For this review, take the finished solid that the model builds, in its own axes (mm). A direction names the side the tool comes from. Round coordinates to 2 decimals unless told otherwise and drop trailing zeros. Write each loop counter-clockwise with the first axis right and the second up, starting at its lowest first coordinate (ties: lowest second). Pieces come first, ordered by that corner, then holes. Notation, with made-up numbers: (87, 28) - (129, 28) arc R15 cw to (129, 33) - close; hole circle Ø3 at (55, 86). An arc over 180 degrees is marked (long way). Answer in a Markdown table with one row per item. Add a question column.
from build123d import *

# Parameters (mm, degrees)
EXTRUDE_1_DEPTH              = 300
HOLE_WIZARD_M6_1_D           = 6.4
HOLE_WIZARD_M6_1_CBORE_D     = 11
HOLE_WIZARD_M6_1_CBORE_DEPTH = 6
CHAMFER_1_SIZE               = 1
CHAMFER_2_SIZE               = 1


with BuildPart() as part:
    # 草图1 → 凸台-拉伸1 (new body)
    with BuildSketch(Plane.XY):
        Polygon((25, 440), (13, 440), (13, 450), (0, 450), (0, 465), (25, 465), align=None)
    extrude(amount=-EXTRUDE_1_DEPTH)

    # M6 凹头盖螺钉的柱形沉头孔1 (through all)
    with Locations(Plane(origin=(25, 0, 0), x_dir=(0, 0, -1), z_dir=(1, 0, 0))):
        with Locations((25, 457.5), (275, 457.5), (150, 457.5)):
            CounterBoreHole(HOLE_WIZARD_M6_1_D / 2, HOLE_WIZARD_M6_1_CBORE_D / 2, HOLE_WIZARD_M6_1_CBORE_DEPTH)

    # 倒角1
    chamfer_1_edges = [part.edges().sort_by_distance(p)[0] for p in [
        (25, 440, -150),
        (13, 440, -150),
        (19, 440, -300),
        (19, 440, 0),
    ]]
    chamfer(chamfer_1_edges, length=CHAMFER_1_SIZE)

    # 倒角2
    chamfer_2_edges = [part.edges().sort_by_distance(p)[0] for p in [
        (25, 465, -150),
    ]]
    chamfer(chamfer_2_edges, length=CHAMFER_2_SIZE)


solid = part.part
Q1. Add section A-A on y = 457.5. State the section outline as (x, z) points.
Q2. Insertion check: pin 1 Ø6.5 at (y, z) = (457.5, -25) entering from -X; pin 2 Ø5 at (y, z) = (444, -161) entering from -X; pin 3 Ø6.5 at (y, z) = (457.5, -275) entering from +X; pin 4 Ø1.5 at (x, z) = (13, -41) entering from -Y. Each pin has a flat end and moves straight along its axis. Give the tip position at first contact, or say it passes through.
Q3. Tool access review of faces 1 (the face through (19, 455.1, -277.4)), 2 (the face through (12, 465, -148)), 3 (the face through (13, 445, -148)): name each direction out of +Z, -Z, +X, -X, +Y, -Y from which nothing blocks a thin tool from reaching the whole face with its end or side.
Q4. Add section C-C on x = 6.5. State the section outline as (y, z) points.
Q5. Add section B-B on z = -150. State the section outline as (x, y) points.
Q6. Add section D-D on z = -233. State the section outline as (x, y) points, then the cut area to 4 significant figures.
Q7. To check wall thickness, follow probe 1 along Z at (x, y) = (22.35, 457.5); probe 2 along Y at (x, z) = (7.5, -275); probe 3 along X at (y, z) = (453.75, -28). State the ranges of each line that lie inside material, in increasing order.
Answer sheet:
| question | item | result |
|---|---|---|
| 1 | outline | (0, -300) - (25, -300) - (25, -280.5) - (19, -280.5) - (19, -278.2) - (0, -278.2) - close; (0, -271.8) - (19, -271.8) - (19, -269.5) - (25, -269.5) - (25, -155.5) - (19, -155.5) - (19, -153.2) - (0, -153.2) - close; (0, -146.8) - (19, -146.8) - (19, -144.5) - (25, -144.5) - (25, -30.5) - (19, -30.5) - (19, -28.2) - (0, -28.2) - close; (0, -21.8) - (19, -21.8) - (19, -19.5) - (25, -19.5) - (25, 0) - (0, 0) - close |
| 2 | pin 1 | stops at x = 0 |
| 2 | pin 2 | stops at x = 13 |
| 2 | pin 3 | stops at x = 19 |
| 2 | pin 4 | stops at y = 440.25 |
| 3 | face 1 | +X |
| 3 | face 2 | +Z, -Z, +X, -X, +Y |
| 3 | face 3 | +Z, -Z, -X, -Y |
| 4 | outline | (450, -300) - (465, -300) - (465, 0) - (450, 0) - close; hole circle Ø6.4 at (457.5, -275); hole circle Ø6.4 at (457.5, -150); hole circle Ø6.4 at (457.5, -25) |
| 5 | outline | (0, 450) - (13, 450) - (13, 441) - (14, 440) - (24, 440) - (25, 441) - (25, 452) - (19, 452) - (19, 454.3) - (0, 454.3) - close; (0, 460.7) - (19, 460.7) - (19, 463) - (25, 463) - (25, 464) - (24, 465) - (0, 465) - close |
| 6 | outline | (0, 450) - (13, 450) - (13, 441) - (14, 440) - (24, 440) - (25, 441) - (25, 464) - (24, 465) - (0, 465) - close |
| 6 | area | 493.5 mm² |
| 7 | probe 1 | z = -300 to -280.5, -269.5 to -155.5, -144.5 to -30.5, -19.5 to 0 |
| 7 | probe 2 | y = 450 to 454.3, 460.7 to 465 |
| 7 | probe 3 | x = 0 to 19 |
